from build123d import *

# Parameters (mm, degrees)
F1_DEPTH = 25.4


with BuildPart() as f1:
    # F0 (on Top) → F1 (new body)
    with BuildSketch(Plane.XY):
        Polygon((72.832607, -21.866195), (72.832607, -177.441195), (101.407607, -21.866195), align=None)
        Polygon((72.832607, 143.233805), (101.407607, 143.233805), (72.832607, 298.808805), align=None)
        with BuildLine():
            Line((-368.492393, -177.441195), (72.832607, -177.441195))
            Line((72.832607, -177.441195), (72.832607, -21.866195))
            Line((72.832607, -21.866195), (72.832607, -10.706964))
            ThreePointArc((72.832607, -10.706964), (62.415429, -16.634584), (50.607607, -18.691195))
            Line((50.607607, -18.691195), (50.607607, 140.058805))
            Line((50.607607, 140.058805), (60.132607, 140.058805))
            ThreePointArc((60.132607, 140.058805), (66.706611, 139.193321), (72.832607, 136.65585))
            Line((72.832607, 136.65585), (72.832607, 143.233805))
            Line((72.832607, 143.233805), (72.832607, 298.808805))
            Line((72.832607, 298.808805), (-368.492393, 298.808805))
            Line((-368.492393, 298.808805), (-368.492393, -177.441195))
        make_face()
        with BuildLine():
            Line((72.832607, -10.706964), (72.832607, -21.866195))
            Line((72.832607, -21.866195), (101.407607, -21.866195))
            Line((101.407607, -21.866195), (101.407607, 143.233805))
            Line((101.407607, 143.233805), (72.832607, 143.233805))
            Line((72.832607, 143.233805), (72.832607, 136.65585))
            ThreePointArc((72.832607, 136.65585), (82.129653, 127.358805), (85.532607, 114.658805))
            Line((85.532607, 114.658805), (85.532607, 16.233805))
            ThreePointArc((85.532607, 16.233805), (82.198459, 1.341735), (72.832607, -10.706964))
        make_face()
    extrude(amount=F1_DEPTH)


solid = f1.part
Design review of the part built by this model. Coordinates are the model's own, in mm. A direction names the side the tool comes from. Round coordinates to 2 decimals unless told otherwise and drop trailing zeros. Order: outer loops, then holes, each group sorted by start corner. A loop starts at its lowest first (then second) coordinate and runs counter-clockwise, first axis right, second up.
1) Consider section A-A (y = 95.5). State the section outline as (x, z) points.
The answers:
outline: (-368.49, 0) - (50.61, 0) - (50.61, 25.4) - (-368.49, 25.4) - close; (85.53, 0) - (101.41, 0) - (101.41, 25.4) - (85.53, 25.4) - close
2) For L1, parallel to X at y = 18.5, z = 16.75; L2, parallel to Y at x = 51, z = 17.25; L3, parallel to X at y = 125.5, z = 23.75, list the stretches that pass through material, from the lowest coordinate up.
The answers:
L1: x = -368.49 to 50.61, 85.53 to 101.41
L2: y = -177.44 to -18.69, 140.06 to 298.81
L3: x = -368.49 to 50.61, 83.1 to 101.41
3) Draft analysis for pull direction X (two halves, no side actions). For faces 1 (the flat face through (-137, 64, 0)), 2 (the flat face through (-368.492, 64, 13)), 3 (the flat face through (85.533, 66, 13)), state which applies: released by +X, released by -X, zero draft, split by the parting line, or undercut.
The answers:
face 1: zero draft
face 2: released by -X
face 3: undercut
4) Consider section B-B (z = 8.25). State the section outline as (x, y) points (3 decimals), plus the area to 3 significant figures.
The answers:
outline: (-368.492, -177.441) - (72.833, -177.441) - (101.408, -21.866) - (101.408, 143.234) - (72.833, 298.809) - (-368.492, 298.809) - close; hole (50.608, -18.691) arc R34.925 ccw to (72.833, -10.707) arc R34.925 ccw to (85.533, 16.234) - (85.533, 114.659) arc R25.4 ccw to (72.833, 136.656) arc R25.4 ccw to (60.133, 140.059) - (50.608, 140.059) - close
area: 214,000 mm2
5) Consider section C-C (y = 206). State the section outline as (x, z) points, plus the area to 3 significant figures.
The answers:
outline: (-368.49, 0) - (89.88, 0) - (89.88, 25.4) - (-368.49, 25.4) - close
area: 11,600 mm2
6) Consider section D-D (y = -86). State the section outline as (x, z) points, plus the area to 3 significant figures.
The answers:
outline: (-368.49, 0) - (89.63, 0) - (89.63, 25.4) - (-368.49, 25.4) - close
area: 11,600 mm2
7) Machinability: for faces 4 (the flat face through (50.608, 60, 13)), 5 (the flat face through (-137, 64, 25.4)), which of the approach directions +Z, -Z, +X, -X, +Y, -Y give a long, thin tool a straight path to every point of the face, cutting with its end or side? Answer none if there is none.
The answers:
face 4: +Z, -Z
face 5: +Z, +X, -X, +Y, -Y
8) Clearance check with a flat-ended pin moving along its axis: pin 1 Ø12 at (y, z) = (-115.5, 3.5) entering from +X. State where the tip first meets the part, or that it passes through.
The answers:
pin 1: stops at x = 85.31
